```python
from build123d import *

# Parameters (mm, degrees)
CYLINDER018_R           = 7
CYLINDER018_DEPTH       = 30
CYLINDER018_PITCH_ANGLE = 90
BOX003_W                = 30
BOX003_H                = 15
BOX003_DEPTH            = 10


with BuildPart() as cylinder018:
    # Cylinder018 → Cylinder018 (new body)
    with BuildSketch(Plane.XY):
        Circle(CYLINDER018_R)
    extrude(amount=CYLINDER018_DEPTH)


with BuildPart() as cylinder018_1:
    # Cylinder018 pitch: moved
    add(cylinder018.part.rotate(Axis((0, 0, 0), (0, 1, 0)), CYLINDER018_PITCH_ANGLE))


with BuildPart() as cylinder018_2:
    # Cylinder018 placement: moved
    add(cylinder018_1.part.moved(Location((0, 0, 13))))


with BuildPart() as cut013:
    # Box003 → Box003 (new body)
    with BuildSketch(Plane(origin=(0, -7, 13), x_dir=(1, 0, 0), z_dir=(0, 0, 1))):
        with Locations((15, 7.5)):
            Rectangle(BOX003_W, BOX003_H)
    extrude(amount=BOX003_DEPTH)

    # Cut013: cut Cylinder018
    add(cylinder018_2.part, mode=Mode.SUBTRACT)


solid = cut013.part
```
Build history of the part. All positions in model axes, mm. Coordinates: 2 decimals unless noted, no trailing zeros. Order: outer loops, then holes, each group sorted by start corner. A loop starts at its lowest first (then second) coordinate and runs counter-clockwise, first axis right, second up.
Item 1: Drill centre lines: L1, parallel to Y at x = 21.5, z = 19; L2, parallel to Y at x = 19.75, z = 15.75; L3, parallel to Z at x = 10.25, y = -1. Where is each one in solid material? Low to high.
Filled in:
L1: y = -7 to -3.61, 3.61 to 8
L2: y = -7 to -6.44, 6.44 to 8
L3: z = 19.93 to 23
Item 2: Saw through at B-B on x = 5.75. List the corners of the cut face in (y, z), then the cut area to 3 significant figures.
Filled in:
outline: (-7, 13) arc R7 cw to (7, 13) - (8, 13) - (8, 23) - (-7, 23) - close
area: 73.0 mm2
Item 3: Saw through at A-A on z = 15.5. List the corners of the cut face in (x, y).
Filled in:
outline: (0, -7) - (30, -7) - (30, -6.54) - (0, -6.54) - close; (0, 6.54) - (30, 6.54) - (30, 8) - (0, 8) - close
Item 4: Saw through at D-D on y = 0. List the corners of the cut face in (x, z), then the cut area to 3 significant figures.
Filled in:
outline: (0, 20) - (30, 20) - (30, 23) - (0, 23) - close
area: 90.0 mm2
Item 5: Drop a flat-ended pin along its axis: pin 1 Ø5 at (x, y) = (19, -0.5) entering from -Z. Give the stop position or say it passes through.
Filled in:
pin 1: stops at z = 19.32
Item 6: Saw through at C-C on z = 19. List the corners of the cut face in (x, y), then the cut area to 3 significant figures.
Filled in:
outline: (0, -7) - (30, -7) - (30, -3.61) - (0, -3.61) - close; (0, 3.61) - (30, 3.61) - (30, 8) - (0, 8) - close
area: 234 mm2
